```python
from build123d import *

# Parameters (mm, degrees)
SKETCH1_R                = 3.5
SKETCH1_R_2              = 1.5
BOSS_EXTRUDE2_DEPTH      = 13.5
CUT_EXTRUDE4_DEPTH       = 70.616522229
CUT_EXTRUDE4_DEPTH_BACK  = 70.616522229
BOSS_EXTRUDE3_DEPTH      = 13
BOSS_EXTRUDE3_DEPTH_BACK = 5
SKETCH4_R                = 6.75
SKETCH7_R                = 1.5
SKETCH7_R_2              = 0.7
BOSS_EXTRUDE4_DEPTH      = 10
SKETCH9_R                = 2.5
BOSS_EXTRUDE5_DEPTH      = 18


with BuildPart() as part:
    # Sketch1 → Boss-Extrude2 (new body)
    with BuildSketch(Plane.XY):
        with BuildLine():
            ThreePointArc((49.948019617, -8.004321858), (65.942252812, 0), (49.948019617, 8.004321858))
            add(Edge.make_bspline(
                [(49.948019617, 8.004321858), (35.174968068, -0.699990604), (18.85115398, 7.452401894)],
                knots=[0, 0, 0, 1, 1, 1], degree=2))
            ThreePointArc((18.85115398, 7.452401894), (7.942252812, 0), (18.85115398, -7.452401894))
            add(Edge.make_bspline(
                [(49.948019617, -8.004321858), (35.174968068, 0.699990604), (18.85115398, -7.452401894)],
                knots=[0, 0, 0, 1, 1, 1], degree=2))
        make_face()
        with Locations((55.942252812, 0)):
            Circle(SKETCH1_R, mode=Mode.SUBTRACT)
        with Locations((15.942252812, 0)):
            Circle(SKETCH1_R_2, mode=Mode.SUBTRACT)
    extrude(amount=BOSS_EXTRUDE2_DEPTH)

    # Sketch3 → Cut-Extrude4 (cut, two sides: drawn at the far end of the back side and taken through both)
    with BuildSketch(Plane(origin=(-0.424036019, 6.116012378, 0), x_dir=(0.9976051599790391, 0.06916606670323111, 0), z_dir=(-0.06916606670323111, 0.9976051599790391, 0)).offset(-CUT_EXTRUDE4_DEPTH_BACK)):
        with BuildLine():
            Line((26.011787518, -9.75), (7.904073667, -9.75))
            Line((7.904073667, -9.75), (7.904073667, -3.75))
            Line((7.904073667, -3.75), (26.011787518, -3.75))
            ThreePointArc((26.011787518, -3.75), (29.011787518, -6.75), (26.011787518, -9.75))
        make_face()
    extrude(amount=CUT_EXTRUDE4_DEPTH + CUT_EXTRUDE4_DEPTH_BACK, mode=Mode.SUBTRACT)

    # Sketch4 → Boss-Extrude3 (add, two sides: drawn at the far end of the back side and taken through both)
    with BuildSketch(Plane(origin=(12.882354757, -29.627387579, 0), x_dir=(0, 0, -1), z_dir=(0.39874906892524703, -0.9170600743851237, 0)).offset(-BOSS_EXTRUDE3_DEPTH_BACK)):
        with Locations(Location((-6.75, 51.958012611, 0), (0, 0, 90))):
            Circle(SKETCH4_R)
    extrude(amount=BOSS_EXTRUDE3_DEPTH + BOSS_EXTRUDE3_DEPTH_BACK)

    # Sketch7 → Boss-Extrude4 (add)
    with BuildSketch(Plane(origin=(18.066092653, -41.549168546, 0), x_dir=(0.9170600743851237, 0.39874906892524703, 0), z_dir=(0.39874906892524703, -0.9170600743851237, 0))):
        with Locations((51.958012611, 6.75)):
            Circle(SKETCH7_R)
        with Locations((51.958012611, 6.75)):
            Circle(SKETCH7_R_2, mode=Mode.SUBTRACT)
    extrude(amount=BOSS_EXTRUDE4_DEPTH)

    # Sketch9 → Boss-Extrude5 (add)
    with BuildSketch(Plane(origin=(18.066092653, -41.549168546, 0), x_dir=(0.9170600743851237, 0.39874906892524703, 0), z_dir=(0.39874906892524703, -0.9170600743851237, 0))):
        with Locations(Location((51.958012611, 6.75, 0), (0, 0, 180))):
            Circle(SKETCH9_R)
    extrude(amount=BOSS_EXTRUDE5_DEPTH)


solid = part.part
```
Source: CAD feature listing. Evaluate the final solid. Frame: model axes, mm. A direction names the side the tool comes from. Coordinates: 2 decimals unless noted, no trailing zeros. Loops run counter-clockwise (first coordinate to the right, second up) from the corner with the lowest first, then second, coordinate; pieces in that order, holes last. Notation, with made-up numbers: (18.5, 42) -> (47.5, 42) arc R23 cw to (47.5, 75) -> close; hole circle Ø8 at (73.5, 13.25). An arc over 180 degrees is marked (long way). One line per item, written item: value. Start each with the question number.
Q1. Section query A-A, the plane x = 12. Return the cut outline in (y, z).
Q2. Set-up query: faces 1 (the face through (17.373, 0.451, 11.599)), 2 (the face through (65.628, -20.869, 3.844)). Return all of +Z, -Z, +X, -X, +Y, -Y with unobstructed straight access to the full face (end or side cutting, diameter ignored); none if empty.
Q3. Section query B-B, the plane y = 0. Give the number of separate pieces and of enclosed holes in the cut face, and give its area (3 significant figures).
Q4. Mould query, pull axis X, two halves, no side actions, for faces 3 (the face through (7.945, 0.218, 1.849)), 4 (the face through (29.065, 0.231, 6.684)), 5 (the face through (17, -2, 9.75)). Classes: pulls with the +X half, pulls with the -X half, needs draft (parallel to the pull), parting line crosses it, or undercut.
Q5. Contact query for flat-ended pins moving along their axis: P1, Ø3, axis at x = 50, z = 1.5, coming from the -Y side; P2, Ø3, axis at x = 62.5, z = 10, coming from the -Y side; P3, Ø1.5, axis at x = 51, z = 7.5, coming from the -Y side; P4, Ø1, axis at x = 51, y = -10, coming from the +Z side. Output: stop coordinate, or through.
Q6. Line query: line 1 along Z through (x, y) = (21, 1); line 2 along Y through (x, z) = (70, 5.5); line 3 along X through (y, z) = (7, 3.5). Output: solid intervals per line, ascending.
Results:
1. outline: (-6.96, 0) -> (6.96, 0) -> (6.96, 3.75) -> (-6.96, 3.75) -> close; (-6.96, 9.75) -> (6.96, 9.75) -> (6.96, 13.5) -> (-6.96, 13.5) -> close
2. face 1: +Z, -Z
2. face 2: none
3. separate pieces: 4
3. enclosed holes: 0
3. area: 543 mm^2
4. face 3: undercut
4. face 4: pulls with the -X half
4. face 5: needs draft
5. P1: y = -8.96
5. P2: y = -22.88
5. P3: y = -9.08
5. P4: through
6. line 1: 0 to 3.75, 9.75 to 13.5
6. line 2: -36.12 to -25.26, -18.97 to -14.05
6. line 3: 12.07 to 19.78, 48.13 to 63.08
